Input: part model. Units: mm. Frame: model coordinates. Face numbers are marked on the shaded views. A direction names the side the tool comes from. Coordinates: 2 decimals unless noted, no trailing zeros. Order: outer loops, then holes, each group sorted by start corner. A loop starts at its lowest first (then second) coordinate and runs counter-clockwise, first axis right, second up. Notation, with made-up numbers: (29.25, -29.75) - (38.25, -29.75) arc R29 cw to (38.25, -3.75) - close; hole circle Ø6 at (-36, 84.5). An arc over 180 degrees is marked (long way). Use a Markdown table: item, result. Add a question column.
from build123d import *

# Parameters (mm, degrees)
BOSS_EXTRUDE1_DEPTH = 7
BOSS_EXTRUDE2_DEPTH = 7
SKETCH3_R           = 1.2
SKETCH3_W           = 3
SKETCH3_H           = 6
SKETCH3_W_2         = 1
SKETCH3_H_2         = 1.756233336
CUT_EXTRUDE1_DEPTH  = 7
CUT_EXTRUDE2_DEPTH  = 2
CUT_EXTRUDE3_START  = -2
CUT_EXTRUDE3_DEPTH  = 2
FILLET1_R           = 2
FILLET2_R           = 1


with BuildPart() as part:
    # Sketch1 → Boss-Extrude1 (new body)
    with BuildSketch(Plane(origin=(0, 0, 0), x_dir=(1, 0, 0), z_dir=(0, 1, 0))):
        with BuildLine():
            ThreePointArc((-3.91606346, 1.893923699), (-4.018875966, 1.664672931), (-4.108281319, 1.429868737))
            ThreePointArc((-4.108281319, 1.429868737), (-4.280699455, 1.194070126), (-4.55544348, 1.094849567))
            ThreePointArc((-4.55544348, 1.094849567), (-5.227650928, 1.004963027), (-5.875844758, 0.805495733))
            ThreePointArc((-5.875844758, 0.805495733), (-6.095335918, 0.633837197), (-6.188868421, 0.371359211))
            ThreePointArc((-6.188868421, 0.371359211), (-6.2, 0), (-6.188868421, -0.371359211))
            ThreePointArc((-6.188868421, -0.371359211), (-6.095335918, -0.633837197), (-5.875844758, -0.805495733))
            ThreePointArc((-5.875844758, -0.805495733), (-5.227650928, -1.004963027), (-4.55544348, -1.094849567))
            ThreePointArc((-4.55544348, -1.094849567), (-4.280699455, -1.194070126), (-4.108281319, -1.429868737))
            ThreePointArc((-4.108281319, -1.429868737), (-4.018875966, -1.664672931), (-3.91606346, -1.893923699))
            ThreePointArc((-3.91606346, -1.893923699), (-3.871246696, -2.182576529), (-3.995360529, -2.447009422))
            ThreePointArc((-3.995360529, -2.447009422), (-4.407123592, -2.985891249), (-4.724421169, -3.585278179))
            ThreePointArc((-4.724421169, -3.585278179), (-4.758243941, -3.861862781), (-4.638781445, -4.113600212))
            ThreePointArc((-4.638781445, -4.113600212), (-4.274116248, -4.491317212), (-3.87880163, -4.836827257))
            ThreePointArc((-3.87880163, -4.836827257), (-3.119853719, -4.489348414), (-2.447009422, -3.995360529))
            ThreePointArc((-2.447009422, -3.995360529), (-2.182576529, -3.871246696), (-1.893923699, -3.91606346))
            ThreePointArc((-1.893923699, -3.91606346), (-1.664672931, -4.018875966), (-1.429868737, -4.108281319))
            ThreePointArc((-1.429868737, -4.108281319), (-1.194070126, -4.280699455), (-1.094849567, -4.55544348))
            ThreePointArc((-1.094849567, -4.55544348), (-1.004963027, -5.227650928), (-0.805495733, -5.875844758))
            ThreePointArc((-0.805495733, -5.875844758), (-0.633837197, -6.095335918), (-0.371359211, -6.188868421))
            ThreePointArc((-0.371359211, -6.188868421), (0, -6.2), (0.371359211, -6.188868421))
            ThreePointArc((0.371359211, -6.188868421), (0.633837197, -6.095335918), (0.805495733, -5.875844758))
            ThreePointArc((0.805495733, -5.875844758), (1.004963027, -5.227650928), (1.094849567, -4.55544348))
            ThreePointArc((1.094849567, -4.55544348), (1.194070126, -4.280699455), (1.429868737, -4.108281319))
            ThreePointArc((1.429868737, -4.108281319), (1.664672931, -4.018875966), (1.893923699, -3.91606346))
            ThreePointArc((1.893923699, -3.91606346), (2.182576529, -3.871246696), (2.447009422, -3.995360529))
            ThreePointArc((2.447009422, -3.995360529), (2.985891249, -4.407123592), (3.585278179, -4.724421169))
            ThreePointArc((3.585278179, -4.724421169), (3.861862781, -4.758243941), (4.113600212, -4.638781445))
            ThreePointArc((4.113600212, -4.638781445), (4.384062043, -4.384062043), (4.638781445, -4.113600212))
            ThreePointArc((4.638781445, -4.113600212), (4.758243941, -3.861862781), (4.724421169, -3.585278179))
            ThreePointArc((4.724421169, -3.585278179), (4.407123592, -2.985891249), (3.995360529, -2.447009422))
            ThreePointArc((3.995360529, -2.447009422), (3.871246696, -2.182576529), (3.91606346, -1.893923699))
            ThreePointArc((3.91606346, -1.893923699), (4.018875966, -1.664672931), (4.108281319, -1.429868737))
            ThreePointArc((4.108281319, -1.429868737), (4.280699455, -1.194070126), (4.55544348, -1.094849567))
            ThreePointArc((4.55544348, -1.094849567), (5.227650928, -1.004963027), (5.875844758, -0.805495733))
            ThreePointArc((5.875844758, -0.805495733), (6.095335918, -0.633837197), (6.188868421, -0.371359211))
            ThreePointArc((6.188868421, -0.371359211), (6.2, 0), (6.188868421, 0.371359211))
            ThreePointArc((6.188868421, 0.371359211), (6.095335918, 0.633837197), (5.875844758, 0.805495733))
            ThreePointArc((5.875844758, 0.805495733), (5.227650928, 1.004963027), (4.55544348, 1.094849567))
            ThreePointArc((4.55544348, 1.094849567), (4.280699455, 1.194070126), (4.108281319, 1.429868737))
            ThreePointArc((4.108281319, 1.429868737), (4.018875966, 1.664672931), (3.91606346, 1.893923699))
            ThreePointArc((3.91606346, 1.893923699), (3.871246696, 2.182576529), (3.995360529, 2.447009422))
            ThreePointArc((3.995360529, 2.447009422), (4.407123592, 2.985891249), (4.724421169, 3.585278179))
            ThreePointArc((4.724421169, 3.585278179), (4.758243941, 3.861862781), (4.638781445, 4.113600212))
            ThreePointArc((4.638781445, 4.113600212), (4.384062043, 4.384062043), (4.113600212, 4.638781445))
            ThreePointArc((4.113600212, 4.638781445), (3.861862781, 4.758243941), (3.585278179, 4.724421169))
            ThreePointArc((3.585278179, 4.724421169), (2.985891249, 4.407123592), (2.447009422, 3.995360529))
            ThreePointArc((2.447009422, 3.995360529), (2.182576529, 3.871246696), (1.893923699, 3.91606346))
            ThreePointArc((1.893923699, 3.91606346), (1.664672931, 4.018875966), (1.429868737, 4.108281319))
            ThreePointArc((1.429868737, 4.108281319), (1.194070126, 4.280699455), (1.094849567, 4.55544348))
            ThreePointArc((1.094849567, 4.55544348), (1.004963027, 5.227650928), (0.805495733, 5.875844758))
            ThreePointArc((0.805495733, 5.875844758), (0.633837197, 6.095335918), (0.371359211, 6.188868421))
            ThreePointArc((0.371359211, 6.188868421), (0, 6.2), (-0.371359211, 6.188868421))
            ThreePointArc((-0.371359211, 6.188868421), (-0.633837197, 6.095335918), (-0.805495733, 5.875844758))
            ThreePointArc((-0.805495733, 5.875844758), (-1.004963027, 5.227650928), (-1.094849567, 4.55544348))
            ThreePointArc((-1.094849567, 4.55544348), (-1.194070126, 4.280699455), (-1.429868737, 4.108281319))
            ThreePointArc((-1.429868737, 4.108281319), (-1.664672931, 4.018875966), (-1.893923699, 3.91606346))
            ThreePointArc((-1.893923699, 3.91606346), (-2.182576529, 3.871246696), (-2.447009422, 3.995360529))
            ThreePointArc((-2.447009422, 3.995360529), (-2.985891249, 4.407123592), (-3.585278179, 4.724421169))
            ThreePointArc((-3.585278179, 4.724421169), (-3.861862781, 4.758243941), (-4.113600212, 4.638781445))
            ThreePointArc((-4.113600212, 4.638781445), (-4.384062043, 4.384062043), (-4.638781445, 4.113600212))
            ThreePointArc((-4.638781445, 4.113600212), (-4.758243941, 3.861862781), (-4.724421169, 3.585278179))
            ThreePointArc((-4.724421169, 3.585278179), (-4.407123592, 2.985891249), (-3.995360529, 2.447009422))
            ThreePointArc((-3.995360529, 2.447009422), (-3.871246696, 2.182576529), (-3.91606346, 1.893923699))
        make_face()
    extrude(amount=BOSS_EXTRUDE1_DEPTH)

    # Sketch2 → Boss-Extrude2 (add)
    with BuildSketch(Plane(origin=(0, 7, 0), x_dir=(1, 0, 0), z_dir=(0, 1, 0))):
        with BuildLine():
            Line((4.25, 0), (4.25, -25))
            ThreePointArc((4.25, -25), (0, -29.25), (-4.25, -25))
            Line((-4.25, -25), (-4.25, 0))
            ThreePointArc((-4.25, 0), (0, 4.25), (4.25, 0))
        make_face()
    extrude(amount=-BOSS_EXTRUDE2_DEPTH)

    # Sketch3 → Cut-Extrude1 (cut)
    with BuildSketch(Plane(origin=(0, 7, 0), x_dir=(1, 0, 0), z_dir=(0, 1, 0))):
        with Locations(Location((0, 0, 0), (0, 0, 270))):
            Circle(SKETCH3_R)
        with Locations(Location((0, -25, 0), (0, 0, 270))):
            Circle(SKETCH3_R)
        with Locations((5.75, -1.514144437)):
            Rectangle(SKETCH3_W, SKETCH3_H)
        with Locations((-4.75, -3.636027769)):
            Rectangle(SKETCH3_W_2, SKETCH3_H_2)
    extrude(amount=-CUT_EXTRUDE1_DEPTH, mode=Mode.SUBTRACT)

    # Sketch5 → Cut-Extrude2 (cut)
    with BuildSketch(Plane.XZ):
        with BuildLine():
            Line((-4.25, 4.375785644), (-4.25, 29.25))
            Line((-4.25, 29.25), (4.25, 29.25))
            Line((4.25, 29.25), (4.25, 4.375785644))
            ThreePointArc((4.25, 4.375785644), (0, 6.1), (-4.25, 4.375785644))
        make_face()
    extrude(amount=-CUT_EXTRUDE2_DEPTH, mode=Mode.SUBTRACT)

    # Sketch6 → Cut-Extrude3 (cut)
    with BuildSketch(Plane(origin=(0, 7, 0), x_dir=(1, 0, 0), z_dir=(0, 1, 0)).offset(CUT_EXTRUDE3_START)):
        with BuildLine():
            Line((-4.25, -4.375785644), (-4.25, -29.25))
            Line((-4.25, -29.25), (4.25, -29.25))
            Line((4.25, -29.25), (4.25, -4.375785644))
            ThreePointArc((4.25, -4.375785644), (0, -6.1), (-4.25, -4.375785644))
        make_face()
    extrude(amount=CUT_EXTRUDE3_DEPTH, mode=Mode.SUBTRACT)

    # Fillet1
    fillet1_edges = [part.edges().sort_by_distance(p)[0] for p in [
        (0, 2, 6.1),
        (0, 5, 6.1),
    ]]
    fillet(fillet1_edges, radius=FILLET1_R - 0.0001)  # a hair under: the kernel refuses the full size

    # Fillet2
    fillet2_edges = [part.edges().sort_by_distance(p)[0] for p in [
        (0, 7, 6.1),
        (0, 0, 6.1),
    ]]
    fillet(fillet2_edges, radius=FILLET2_R)


solid = part.part
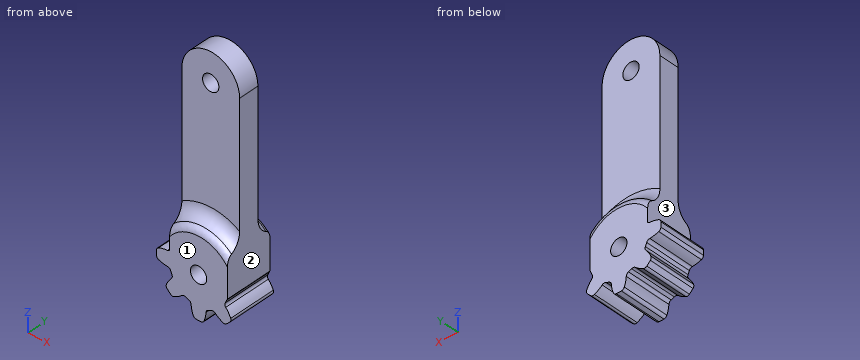
1) Material intervals for L1, parallel to X at y = 3.25, z = 0; L2, parallel to X at y = 3.8, z = 25; L3, parallel to Z at x = 0.75, y = 4.75, sorted ascending.
2) Cut plane B-B (x = 0). State how many separate pieces and enclosed holes the cut face has, and give its area (3 significant figures).
3) Cut plane D-D (z = 20.5). Return the cut outline in (x, y).
4) Reachability of the marked faces 1, 2 and 3 from +Z, -Z, +X, -X, +Y, -Y: full face, straight path, thin tool, end or side. Return the list, or none.
5) Contact query for flat-ended pins moving along their axis: P1, Ø3.5, axis at y = 2, z = 11.5, coming from the -X side; P2, Ø2, axis at x = 3.5, y = 3.5, coming from the +Z side; P3, Ø1.5, axis at x = 3.5, z = 25, coming from the +Y side. Output: stop coordinate, or through.
6) Cut plane A-A (z = 0). Return the cut outline in (x, y).
Computed:
| question | item | result |
|---|---|---|
| 1 | L1 | x = -6.2 to -1.2, 1.2 to 4.25 |
| 1 | L2 | x = -4.25 to -1.2, 1.2 to 4.25 |
| 1 | L3 | z = -5.98 to -0.94, 0.94 to 24.06, 25.94 to 29.18 |
| 2 | separate pieces | 3 |
| 2 | enclosed holes | 0 |
| 2 | area | 133 mm2 |
| 3 | outline | (-4.25, 2) - (4.25, 2) - (4.25, 5) - (-4.25, 5) - close |
| 4 | face 1 | +Z, -Z, +X, -X, -Y |
| 4 | face 2 | +Z, +X, +Y, -Y |
| 4 | face 3 | +Z, -X, +Y, -Y |
| 5 | P1 | stops at x = -4.25 |
| 5 | P2 | stops at z = 28.44 |
| 5 | P3 | stops at y = 5 |
| 6 | outline | (-6.2, 0) - (-1.2, 0) - (-1.2, 7) - (-6.2, 7) - close; (1.2, 0) - (4.25, 0) - (4.25, 7) - (1.2, 7) - close |
